Solid Edge part; units mm, degrees
sketch "Sketch1" plane through (0, 0, 0) normal (0, -1, 0) x (1, 0, 0)
  arc A0 (-67.2, -0.6) -> (-52.8, -0.6) centre (-60, -0.6) cw
  arc A1 (-52.8, -0.6) -> (-43.2, -0.6) centre (-48, -0.6) ccw
  arc A2 (-43.2, -0.6) -> (-28.8, -0.6) centre (-36, -0.6) cw
  arc A3 (-28.8, -0.6) -> (-19.2, -0.6) centre (-24, -0.6) ccw
  arc A4 (-19.2, -0.6) -> (-4.8, -0.6) centre (-12, -0.6) cw
  arc A5 (-4.8, -0.6) -> (4.8, -0.6) centre (0, -0.6) ccw
  arc A6 (4.8, -0.6) -> (19.2, -0.6) centre (12, -0.6) cw
  arc A7 (19.2, -0.6) -> (28.8, -0.6) centre (24, -0.6) ccw
  arc A8 (28.8, -0.6) -> (43.2, -0.6) centre (36, -0.6) cw
  arc A9 (43.2, -0.6) -> (52.8, -0.6) centre (48, -0.6) ccw
  arc A10 (52.8, -0.6) -> (67.2, -0.6) centre (60, -0.6) cw
  arc A11 (67.2, -0.6) -> (76.8, -0.6) centre (72, -0.6) ccw
  arc A12 (76.8, -0.6) -> (91.2, -0.6) centre (84, -0.6) cw
  arc A13 (91.2, -0.6) -> (100.8, -0.6) centre (96, -0.6) ccw
  arc A14 (100.8, -0.6) -> (115.2, -0.6) centre (108, -0.6) cw
  line L0 (114, -0.6) -> (115.2, -0.6)
  arc A15 (102, -0.6) -> (114, -0.6) centre (108, -0.6) cw
  arc A16 (90, -0.6) -> (102, -0.6) centre (96, -0.6) ccw
  arc A17 (78, -0.6) -> (90, -0.6) centre (84, -0.6) cw
  arc A18 (66, -0.6) -> (78, -0.6) centre (72, -0.6) ccw
  arc A19 (54, -0.6) -> (66, -0.6) centre (60, -0.6) cw
  arc A20 (42, -0.6) -> (54, -0.6) centre (48, -0.6) ccw
  arc A21 (30, -0.6) -> (42, -0.6) centre (36, -0.6) cw
  arc A22 (18, -0.6) -> (30, -0.6) centre (24, -0.6) ccw
  arc A23 (6, -0.6) -> (18, -0.6) centre (12, -0.6) cw
  arc A24 (-6, -0.6) -> (6, -0.6) centre (0, -0.6) ccw
  arc A25 (-18, -0.6) -> (-6, -0.6) centre (-12, -0.6) cw
  arc A26 (-30, -0.6) -> (-18, -0.6) centre (-24, -0.6) ccw
  arc A27 (-42, -0.6) -> (-30, -0.6) centre (-36, -0.6) cw
  arc A28 (-54, -0.6) -> (-42, -0.6) centre (-48, -0.6) ccw
  arc A29 (-66, -0.6) -> (-54, -0.6) centre (-60, -0.6) cw
  arc A30 (-78, -0.6) -> (-66, -0.6) centre (-72, -0.6) ccw
  arc A31 (-90, -0.6) -> (-78, -0.6) centre (-84, -0.6) cw
  arc A32 (-102, -0.6) -> (-90, -0.6) centre (-96, -0.6) ccw
  arc A33 (-114, -0.6) -> (-102, -0.6) centre (-108, -0.6) cw
  line L1 (-115.2, -0.6) -> (-114, -0.6)
  arc A34 (-115.2, -0.6) -> (-100.8, -0.6) centre (-108, -0.6) cw
  arc A35 (-100.8, -0.6) -> (-91.2, -0.6) centre (-96, -0.6) ccw
  arc A36 (-91.2, -0.6) -> (-76.8, -0.6) centre (-84, -0.6) cw
  arc A37 (-76.8, -0.6) -> (-67.2, -0.6) centre (-72, -0.6) ccw
extrude "Protrusion1" add sketch "Sketch1" against normal blind 230
Design review of the part built by this model. Coordinates are the model's own, in mm. Coordinates: 2 decimals unless noted, no trailing zeros. Order: outer loops, then holes, each group sorted by start corner. A loop starts at its lowest first (then second) coordinate and runs counter-clockwise, first axis right, second up.
1) Take a section at C-C, the plane x = 37.5. Give the boundary of the cut face in (y, z).
2) Wall thickness on line 1 along Z through (x, y) = (-11.5, 12); line 2 along Z through (x, y) = (-73.5, 103): over which ranges is each line inside the solid? List them lowest first.
3) Take a section at A-A, the plane z = -2.75. State how many separate pieces and enclosed holes the cut face has, and give its area (3 significant figures).
4) Take a section at B-B, the plane x = -24. Give the boundary of the cut face in (y, z).
5) Clearance check with flat-ended pins moving along their axes: pin 1 (6 mm diameter, centred on y = 80.5, z = 4, fed in from -X); pin 2 (3 mm diameter, centred on x = 31.5, y = 146.5, fed in from +Z); pin 3 (1 mm diameter, centred on x = -114.5, y = 114.5, fed in from -Z); pin 4 (8 mm diameter, centred on x = 47.5, y = 182.5, fed in from -Z). State where each tip first meets the part, or that it passes through.
6) Mouldability with a two-part tool opening along X and no side actions: class faces 1 (the flat face through (1, 230, -6)), 2 (the cylindrical face through (23.9, 113.4, -5.4)) as +X half, -X half, draft (parallel to the pull), parting line (faces both ways), or undercut.
Returned:
1. outline: (0, 5.21) - (230, 5.21) - (230, 6.44) - (0, 6.44) - close
2. line 1: z = 5.38 to 6.58
2. line 2: z = -6.41 to -5.16
3. separate pieces: 18
3. enclosed holes: 0
3. area: 5,420 mm2
4. outline: (0, -6.6) - (230, -6.6) - (230, -5.4) - (0, -5.4) - close
5. pin 1: stops at x = -115.02
5. pin 2: stops at z = 5.95
5. pin 3: stops at z = -0.6
5. pin 4: stops at z = -6.6
6. face 1: draft
6. face 2: undercut
